from build123d import *

# Parameters (mm, degrees)
SKETCH020_R             = 11.75
SKETCH020_R_2           = 9.25
PAD014_DEPTH            = 70
SKETCH021_W             = 31.48
SKETCH021_H             = 3
POCKET004_DEPTH         = 67
CHAMFER005_SIZE         = 2
SKETCH022_W             = 3
SKETCH022_H             = 31.59
POCKET005_DEPTH         = 67
BODY012_PLACEMENT_ANGLE = 180


with BuildPart() as part:
    # Sketch020 → Pad014 (new body)
    with BuildSketch(Plane.XY):
        Circle(SKETCH020_R)
        Circle(SKETCH020_R_2, mode=Mode.SUBTRACT)
    extrude(amount=PAD014_DEPTH)

    # Sketch021 (on Face3 of Pad014) → Pocket004 (cut)
    with BuildSketch(Plane(origin=(0, 0, 0), x_dir=(1, 0, 0), z_dir=(0, 0, -1))):
        Rectangle(SKETCH021_W, SKETCH021_H)
    extrude(amount=-POCKET004_DEPTH, mode=Mode.SUBTRACT)

    # Chamfer005
    chamfer005_edges = [part.edges().sort_by_distance(p)[0] for p in [
        (0, 11.75, 0),
        (0, -11.75, 0),
    ]]
    chamfer(chamfer005_edges, length=CHAMFER005_SIZE)

    # Sketch022 (on Face11 of Chamfer005) → Pocket005 (cut)
    with BuildSketch(Plane(origin=(0, 0, 0), x_dir=(1, 0, 0), z_dir=(0, 0, -1))):
        Rectangle(SKETCH022_W, SKETCH022_H)
    extrude(amount=-POCKET005_DEPTH, mode=Mode.SUBTRACT)


with BuildPart() as part_1:
    # Body012 placement: moved
    add(part.part.moved(Location((0, 0, 69))).rotate(Axis((0, 0, 69), (1, 0, 0)), BODY012_PLACEMENT_ANGLE))


solid = part_1.part
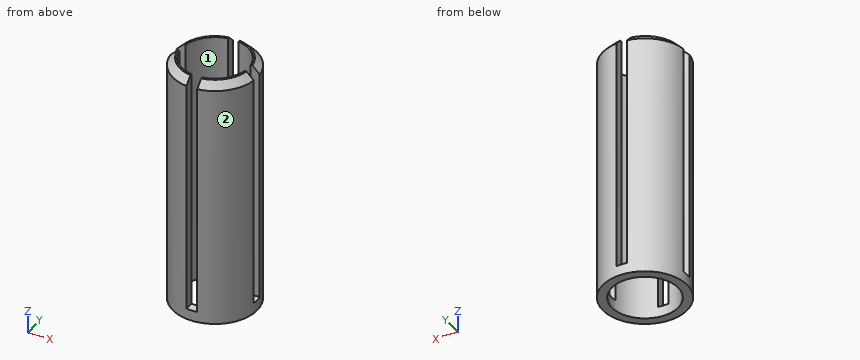
The listing builds one solid part. Answer for the finished solid, in the listing's coordinates (mm). Face numbers are marked on the shaded views. Coordinates: 2 decimals unless noted, no trailing zeros. Write each loop counter-clockwise with the first axis right and the second up, starting at its lowest first coordinate (ties: lowest second). Pieces come first, ordered by that corner, then holes. Notation, with made-up numbers: (66.25, 54) - (109.25, 54) arc R16 cw to (109.25, 64) - close; hole circle Ø1 at (63.5, 56). An arc over 180 degrees is marked (long way). Put each result on its own line as item: value.
1. Determine the mould class of the marked faces 1 and 2 for opening direction X: pulls with the +X half, pulls with the -X half, needs draft (parallel to the pull), parting line crosses it, or undercut.
Answer sheet:
face 1: undercut
face 2: parting line crosses it
2. The part is cut by section A-A on x = 0. Give the vertices of the cut face in (y, z), plus the area to 3 significant figures.
Answer sheet:
outline: (-11.75, -1) - (-9.25, -1) - (-9.25, 2) - (-11.75, 2) - close; (9.25, -1) - (11.75, -1) - (11.75, 2) - (9.25, 2) - close
area: 15.0 mm^2
3. Find the intervals of material crossed by line 1 along Y through (x, z) = (10, 31); line 2 along Y through (x, z) = (-2.5, 17.5); line 3 along X through (y, z) = (7, 40.5), in increasing order. Write a range as from..to.
Answer sheet:
line 1: y = -6.17..-1.5, 1.5..6.17
line 2: y = -11.48..-8.91, 8.91..11.48
line 3: x = -9.44..-6.05, 6.05..9.44
4. Flat-ended cylindrical pins translate along their axes: pin 1 Ø1.3 at (y, z) = (10, 20) entering from +X; pin 2 Ø2 at (x, z) = (7, 18) entering from -Y; pin 3 Ø1.3 at (x, y) = (0, -10) entering from +Z. Find the tip coordinate at first contact, or state that the pin passes through.
Answer sheet:
pin 1: stops at x = 7.12
pin 2: stops at y = -10.1
pin 3: stops at z = 2
5. The part is cut by section B-B on z = 49.5. Give the vertices of the cut face in (x, y), plus the area to 3 significant figures.
Answer sheet:
outline: (-11.65, -1.5) arc R11.75 ccw to (-1.5, -11.65) - (-1.5, -9.13) arc R9.25 cw to (-9.13, -1.5) - close; (-11.65, 1.5) - (-9.13, 1.5) arc R9.25 cw to (-1.5, 9.13) - (-1.5, 11.65) arc R11.75 ccw to start; (1.5, -11.65) arc R11.75 ccw to (11.65, -1.5) - (9.13, -1.5) arc R9.25 cw to (1.5, -9.13) - close; (1.5, 9.13) arc R9.25 cw to (9.13, 1.5) - (11.65, 1.5) arc R11.75 ccw to (1.5, 11.65) - close
area: 135 mm^2
